Design review of the part built by this model. Coordinates are the model's own, in mm. Round coordinates to 2 decimals unless told otherwise and drop trailing zeros. Loops run counter-clockwise (first coordinate to the right, second up) from the corner with the lowest first, then second, coordinate; pieces in that order, holes last. Notation, with made-up numbers: (84.25, 80.25) -> (141.25, 80.25) arc R8 cw to (141.25, 91.25) -> close; hole circle Ø11 at (40, 29.5). An arc over 180 degrees is marked (long way). Use a Markdown table: item, result. Add a question column.
Autodesk Inventor part; units mm, degrees
ref_plane "YZ Plane" through (0, 0, 0) normal (1, 0, 0) x (0, 1, 0)
ref_plane "XZ Plane" through (0, 0, 0) normal (0, 1, 0) x (-1, 0, 0)
ref_plane "XY Plane" through (0, 0, 0) normal (0, 0, 1) x (1, 0, 0)
sketch "Boceto1" plane through (0, 0, 0) normal (0, 0, 1) x (1, 0, 0)
  line L0 (-75.5202, 28.6978) -> (6.4858, 28.6978)
  line L1 (46.1178, -1.7877) -> (-35.8882, -1.7877)
  line L2 (-75.5202, 28.6978) -> (-35.8882, -1.7877)
  line L3 (-35.8882, -1.7877) -> (-35.8882, -1.7877)
  line L4 (6.4858, 28.6978) -> (31.8808, 9.1636)
  line L5 (31.8808, 9.1636) -> (46.1178, -1.7877)
  line L6 (-35.8882, -1.7877) -> (-20.031, -13.9853)
  point P0 (0, 0)
  point P1 (-35.8882, -1.7877)
  dimension "d3" = 82.006
  dimension "d13" = 37.568
  dimension "d14" = 37.568
  dimension "d15" = 30.4855
extrude "Extrusión1" add sketch "Boceto1" along normal blind 10
properties part number "Brazo_C" material "Hierro, fundido"
1. Consider section B-B on x = -64.5. State the section outline as (y, z) points, plus the area to 3 significant figures.
2. Insertion check: P1, Ø2, axis at x = -60, z = 8.5, coming from the -Y side; P2, Ø1.5, axis at y = 3.5, z = 5.5, coming from the -X side; P3, Ø5, axis at y = 20, z = 1.5, coming from the +X side; P4, Ø2, axis at x = -34, y = 11.5, coming from the -Z side. Each pin has a flat end and moves straight along its axis. Give the tip position at first contact, or say it passes through.
3. Consider section C-C on y = 25. State the section outline as (x, z) points, plus the area to 3 significant figures.
4. To check wall thickness, follow probe 1 along X at (y, z) = (24, 7); probe 2 along X at (y, z) = (9, 9.25); probe 3 along Y at (x, z) = (-70, 1.75). State the ranges of each line that lie inside material, in increasing order. Write a range as from..to.
5. Consider section A-A on z = 3.75. State the section outline as (x, y) points.
Verdict:
| question | item | result |
|---|---|---|
| 1 | outline | (20.22, 0) -> (28.7, 0) -> (28.7, 10) -> (20.22, 10) -> close |
| 1 | area | 84.8 mm² |
| 2 | P1 | stops at y = 15.99 |
| 2 | P2 | stops at x = -43.74 |
| 2 | P3 | stops at x = 21.04 |
| 2 | P4 | stops at z = 0 |
| 3 | outline | (-70.71, 0) -> (11.29, 0) -> (11.29, 10) -> (-70.71, 10) -> close |
| 3 | area | 820 mm² |
| 4 | probe 1 | x = -69.41..12.59 |
| 4 | probe 2 | x = -49.91..32.09 |
| 4 | probe 3 | y = 24.45..28.7 |
| 5 | outline | (-75.52, 28.7) -> (-35.89, -1.79) -> (46.12, -1.79) -> (31.88, 9.16) -> (6.49, 28.7) -> close |
